Check sheet for the modelled part. Datum: model origin and axes. Units: mm. Face numbers are marked on the shaded views. Coordinates: 2 decimals unless noted, no trailing zeros. Loops run counter-clockwise (first coordinate to the right, second up) from the corner with the lowest first, then second, coordinate; pieces in that order, holes last. Notation, with made-up numbers: M 29.5,8.25 L 60.5,8.25 A17 cw 60.5,26.25 Z; hole C 21,3.5 d3. An arc over 180 degrees is marked long. Return JSON: item names as keys, results as strings.
from build123d import *

# Parameters (mm, degrees)
CYLINDER002_R     = 3.15
CYLINDER002_DEPTH = 24
BOX002_W          = 27
BOX002_H          = 14.5
BOX002_DEPTH      = 16
FILLET_R          = 3


with BuildPart() as cylinder002:
    # Cylinder002 → Cylinder002 (new body)
    with BuildSketch(Plane(origin=(-15, 37.5, 25), x_dir=(1, 0, 0), z_dir=(0, 0, 1))):
        Circle(CYLINDER002_R)
    extrude(amount=CYLINDER002_DEPTH)


with BuildPart() as cut002002002007004004001003:
    # Box002 → Box002 (new body)
    with BuildSketch(Plane(origin=(-27, 30.5, 30), x_dir=(1, 0, 0), z_dir=(0, 0, 1))):
        with Locations((13.5, 7.25)):
            Rectangle(BOX002_W, BOX002_H)
    extrude(amount=BOX002_DEPTH)

    # Fillet
    fillet_edges = [cut002002002007004004001003.edges().sort_by_distance(p)[0] for p in [
        (-27, 30.5, 38),
        (-27, 45, 38),
    ]]
    fillet(fillet_edges, radius=FILLET_R)

    # Cut002002002007004004001003: cut Cylinder002
    add(cylinder002.part, mode=Mode.SUBTRACT)


solid = cut002002002007004004001003.part
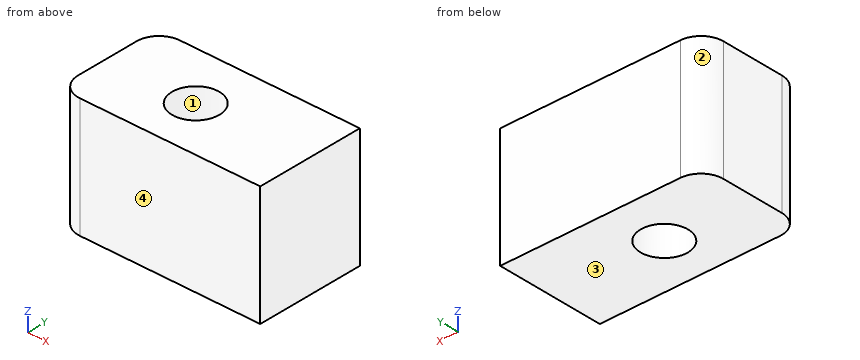
1) Draft check along Y on the marked faces 1, 2, 3 and 4. Enter one of: +Y half, -Y half, draft (parallel to the pull), parting line (faces both ways), or undercut.
Answers:
{"face 1": "undercut", "face 2": "+Y half", "face 3": "draft", "face 4": "-Y half"}
2) Section check A-A on x = -15. Record the cut outline in (y, z), then the cut area to 3 significant figures.
Answers:
{"outline": "M 30.5,30 L 34.35,30 L 34.35,46 L 30.5,46 Z; M 40.65,30 L 45,30 L 45,46 L 40.65,46 Z", "area": "131 mm²"}
3) Section check C-C on y = 37.5. Record the cut outline in (x, z).
Answers:
{"outline": "M -27,30 L -18.15,30 L -18.15,46 L -27,46 Z; M -11.85,30 L 0,30 L 0,46 L -11.85,46 Z"}
4) Go/stop test with a flat-tipped pin: pin 1 Ø5.5 at (x, y) = (-15, 37.5) entering from -Z. Record where the tip stops, or that it passes through.
Answers:
{"pin 1": "through"}
5) Section check B-B on z = 35.25. Record the cut outline in (x, y), then the cut area to 3 significant figures.
Answers:
{"outline": "M -27,33.5 A3 ccw -24,30.5 L 0,30.5 L 0,45 L -24,45 A3 ccw -27,42 Z; hole C -15,37.5 d6.3", "area": "356 mm²"}
6) Scan lines: line 1 along Y through (x, z) = (-15, 42.75); line 2 along X through (y, z) = (37.5, 40.5); line 3 along X through (y, z) = (38.5, 32). Record each from-to range of solid material in increasing order. Write a range as [from, to].
Answers:
{"line 1": "[30.5, 34.35], [40.65, 45]", "line 2": "[-27, -18.15], [-11.85, 0]", "line 3": "[-27, -17.99], [-12.01, 0]"}
